from build123d import *

# Parameters (mm, degrees)
BOSS_EXTRU_7_DEPTH          = 35
BOSS_EXTRU_8_DEPTH          = 5
ESQUISSE3_R                 = 2.5
ENL_V_MAT_EXTRU_1_DEPTH     = 5
ENL_V_MAT_EXTRU_2_DEPTH     = 12
ESQUISSE6_R                 = 9.75
ENL_V_MAT_EXTRU_3_DEPTH     = 5
CONG_1_R                    = 2
ESQUISSE8_R                 = 1.5
ENL_V_MAT_EXTRU_5_DEPTH     = 90.727364834
TROU_TARAUD_M31_D           = 2.5
TROU_TARAUD_M31_DEPTH       = 12.5
TROU_TARAUD_M31_TIP         = 0.751075774
ENL_V_START                 = -35
ENL_V_MAT_EXTRU_6_OUTLINE_R = 1.475
ENL_V_MAT_EXTRU_6_DEPTH     = 10
ENL_V_MAT_EXTRU_7_DEPTH     = 99.692704898
ENL_V_MAT_EXTRU_8_DEPTH     = 10


# Read off the part's stored shape, not the designer's step: Enlèv. mat.-Extru.6
with BuildPart() as part:
    # Esquisse1 → Boss.-Extru.7 (new, symmetric)
    with BuildSketch(Plane(origin=(0, 0, 0), x_dir=(1, 0, 0), z_dir=(0, 1, 0))):
        Polygon((-35, 31), (-35, -31), (0, -31), (0, -26), (-25, -26), (-25, -22.1), (-25, -17.1), (-25, 17.1), (-25, 22.1), (-25, 26), (0, 26), (0, 31), align=None)
    extrude(amount=BOSS_EXTRU_7_DEPTH, both=True)

    # Esquisse2 → Boss.-Extru.8 (add)
    with BuildSketch(Plane.XZ.offset(35)):
        with BuildLine():
            Line((-35, 37.094473982), (-35, -37.094473982))
            ThreePointArc((-35, -37.094473982), (-18.830584523, -47.396298237), (0, -51))
            Line((0, -51), (0, 51))
            ThreePointArc((0, 51), (-18.830584523, 47.396298237), (-35, 37.094473982))
        make_face()
    extrude(amount=-BOSS_EXTRU_8_DEPTH)

    # Esquisse3 → Enlèv. mat.-Extru.1 (cut)
    with BuildSketch(Plane(origin=(-25, 0, 0), x_dir=(0, 0, -1), z_dir=(1, 0, 0))):
        with Locations((-19.6, -2.21)):
            Circle(ESQUISSE3_R)
        with Locations((19.6, -2.21)):
            Circle(ESQUISSE3_R)
    extrude(amount=-ENL_V_MAT_EXTRU_1_DEPTH, mode=Mode.SUBTRACT)

    # Esquisse5 → Enlèv. mat.-Extru.2 (cut)
    with BuildSketch(Plane(origin=(0, 0, 0), x_dir=(0, 0, -1), z_dir=(1, 0, 0))):
        with BuildLine():
            Line((98.051206934, 14.815086571), (40.674477228, 51.032394683))
            ThreePointArc((40.674477228, 51.032394683), (34.260412481, 48.633219758), (27.706013605, 46.649253461))
            ThreePointArc((27.706013605, 46.649253461), (-0.631861598, 43.001865666), (-28.924683694, 46.983677637))
            ThreePointArc((-28.924683694, 46.983677637), (-34.858411147, 48.837303455), (-40.674477228, 51.032394683))
            Line((-40.674477228, 51.032394683), (-98.051206934, 14.815086571))
            ThreePointArc((-98.051206934, 14.815086571), (-66.125172065, -3.350779651), (-31, -14.097531974))
            Line((-31, -14.097531974), (-31, 35))
            Line((-31, 35), (-26, 35))
            Line((-26, 35), (-26, -14.963632356))
            ThreePointArc((-26, -14.963632356), (0, -17), (26, -14.963632356))
            Line((26, -14.963632356), (26, 35))
            Line((26, 35), (31, 35))
            Line((31, 35), (31, -14.097531974))
            ThreePointArc((31, -14.097531974), (66.125172065, -3.350779651), (98.051206934, 14.815086571))
        make_face()
        with BuildLine():
            ThreePointArc((-31, -14.097531974), (-28.503289853, -14.549574498), (-26, -14.963632356))
            Line((-26, -14.963632356), (-26, 35))
            Line((-26, 35), (-31, 35))
            Line((-31, 35), (-31, -14.097531974))
        make_face()
        with BuildLine():
            ThreePointArc((26, -14.963632356), (28.503289853, -14.549574498), (31, -14.097531974))
            Line((31, -14.097531974), (31, 35))
            Line((31, 35), (26, 35))
            Line((26, 35), (26, -14.963632356))
        make_face()
    extrude(amount=-ENL_V_MAT_EXTRU_2_DEPTH, mode=Mode.SUBTRACT)

    # Esquisse6 → Enlèv. mat.-Extru.3 (cut)
    with BuildSketch(Plane(origin=(-25, 0, 0), x_dir=(0, 0, -1), z_dir=(1, 0, 0))):
        with Locations((0, 20)):
            Circle(ESQUISSE6_R)
    extrude(amount=-ENL_V_MAT_EXTRU_3_DEPTH, mode=Mode.SUBTRACT)

    # Congé1
    cong_1_edges = [part.edges().sort_by_distance(p)[0] for p in [
        (-23.5, 35, 31),
        (-18.5, 35, 26),
        (-25, 35, 0),
        (-18.5, 35, -26),
        (-23.5, 35, -31),
        (-12, 35, -28.5),
        (-12, 35, 28.5),
        (-35, 35, 0),
    ]]
    fillet(cong_1_edges, radius=CONG_1_R)

    # Esquisse8 → Enlèv. mat.-Extru.5 (cut, through all)
    with BuildSketch(Plane(origin=(0, -30, 0), x_dir=(1, 0, 0), z_dir=(0, 1, 0))):
        with Locations(Location((-21, 41, 0), (0, 0, 270))):
            Circle(ESQUISSE8_R)
        with Locations(Location((-6, 41, 0), (0, 0, 270))):
            Circle(ESQUISSE8_R)
        with Locations(Location((-6, -41, 0), (0, 0, 90))):
            Circle(ESQUISSE8_R)
        with Locations(Location((-21, -41, 0), (0, 0, 90))):
            Circle(ESQUISSE8_R)
    extrude(amount=-ENL_V_MAT_EXTRU_5_DEPTH, mode=Mode.SUBTRACT)

    # Trou taraudé M31
    with Locations(Plane(origin=(-35, 18, -4), x_dir=(0, 0, -1), z_dir=(-1, 0, 0))):
        with Locations((0, 0), (-15, 0), (-30, 0)):
            Hole(TROU_TARAUD_M31_D / 2, depth=TROU_TARAUD_M31_DEPTH)
            with Locations((0, 0, -(TROU_TARAUD_M31_DEPTH + TROU_TARAUD_M31_TIP / 2))):  # 118° drill point
                Cone(0, TROU_TARAUD_M31_D / 2, TROU_TARAUD_M31_TIP, mode=Mode.SUBTRACT)

    # Enlèv. mat.-Extru.6 outline → Enlèv. mat.-Extru.6 (cut)
    with BuildSketch(Plane.YZ.offset(ENL_V_START)):
        with Locations((10, -14.5)):
            Circle(ENL_V_MAT_EXTRU_6_OUTLINE_R)
        with Locations((10, 14.5)):
            Circle(ENL_V_MAT_EXTRU_6_OUTLINE_R)
    extrude(amount=ENL_V_MAT_EXTRU_6_DEPTH, mode=Mode.SUBTRACT)

    # Esquisse3D3 → Enlèv. mat.-Extru.7 (cut, through all)
    with BuildSketch(Plane(origin=(0, -30, -14.5), x_dir=(-0.586509812151843, 0, 0.8099421215430211), z_dir=(0, -1, 0))):
        Polygon((0, 0), (12.316706055, 17.008784552), (35.80502758, 0), (23.488321525, -17.008784552), align=None)
    extrude(amount=ENL_V_MAT_EXTRU_7_DEPTH, mode=Mode.SUBTRACT)

    # Esquisse3D4 → Enlèv. mat.-Extru.8 (cut)
    with BuildSketch(Plane(origin=(0, -22, -31), x_dir=(-0.8574929257125444, -0.5144957554275261, 0), z_dir=(0, 0, -1))):
        Polygon((0, 0), (4.287464629, 2.572478777), (5.830951895, 0), (1.543487266, -2.572478777), align=None)
    extrude(amount=-ENL_V_MAT_EXTRU_8_DEPTH, mode=Mode.SUBTRACT)


solid = part.part
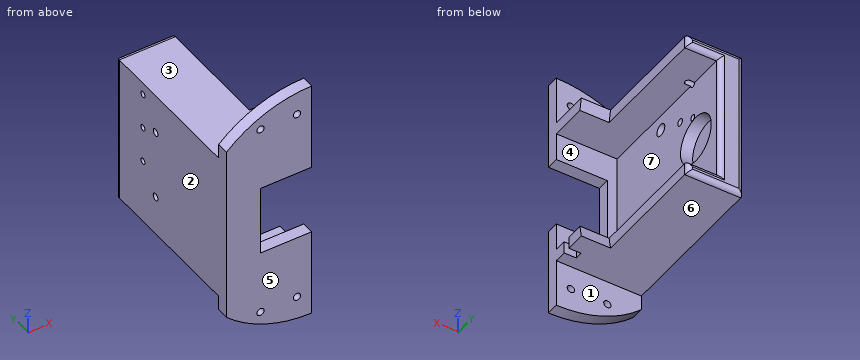
Design review of the part built by this model. Coordinates are the model's own, in mm. Face numbers are marked on the shaded views. A direction names the side the tool comes from. Coordinates: 2 decimals unless noted, no trailing zeros. Loops run counter-clockwise (first coordinate to the right, second up) from the corner with the lowest first, then second, coordinate; pieces in that order, holes last.
Item 1: For the marked faces 1, 2, 3 and 4, list the 3-axis set-ups (+Z, -Z, +X, -X, +Y, -Y) from which the entire face can be reached by the end or side of a thin tool; tool diameter is ignored.
Completed:
face 1: -Z, +X, -X, +Y
face 2: +Z, -Z, -X, +Y, -Y
face 3: +Z, +X, -X, +Y
face 4: +X, +Y
Item 2: Clearance check with flat-ended pins moving along their axes: pin 1 (4 mm diameter, centred on x = -6, z = -41, fed in from +Y); pin 2 (2.5 mm diameter, centred on x = -2, z = -28.5, fed in from +Y); pin 3 (2.5 mm diameter, centred on y = -2.5, z = 19, fed in from +X). State where each tip first meets the part, or that it passes through.
Completed:
pin 1: stops at y = -30
pin 2: stops at y = -14.33
pin 3: stops at x = -30
Item 3: Wall thickness on L1, parallel to Y at x = -28.6, z = 0; L2, parallel to Z at x = -24, y = 18; L3, parallel to Z at x = -32, y = 18: over which ranges is each line inside the solid? List them lowest first.
Completed:
L1: y = -35 to 10.25, 29.75 to 35
L2: z = -31 to -26, 27.25 to 31
L3: z = -31 to -5.25, -2.75 to 9.75, 12.25 to 24.75, 27.25 to 31
Item 4: Add section C-C (z = 41). Write out the cut boundary in (x, y).
Completed:
outline: (-30.33, -35) - (-22.5, -35) - (-22.5, -30) - (-30.33, -30) - close; (-19.5, -35) - (-7.5, -35) - (-7.5, -30) - (-19.5, -30) - close; (-4.5, -35) - (0, -35) - (0, -30) - (-4.5, -30) - close
Item 5: Add section B-B (z = -19.6). Write out the cut boundary in (x, y).
Completed:
outline: (-35, -35) - (0, -35) - (0, -30) - (-25, -30) - (-25, -4.71) - (-30, -4.71) - (-30, 0.29) - (-25, 0.29) - (-25, 33) arc R2 ccw to (-27, 35) - (-33, 35) arc R2 ccw to (-35, 33) - close
Item 6: Add section A-A (y = -8.5). Write out the cut boundary in (x, z).
Completed:
outline: (-35, -31) - (-12, -31) - (-12, -26) - (-25, -26) - (-25, 26) - (-12, 26) - (-12, 31) - (-35, 31) - close
Item 7: Add section D-D (y = 15). Write out the cut boundary in (x, z), and give its area (3 significant figures).
Completed:
outline: (-35, -31) - (-12, -31) - (-12, -26) - (-25, -26) - (-25, -8.37) - (-30, -8.37) - (-30, 8.37) - (-25, 8.37) - (-25, 26) - (-12, 26) - (-12, 31) - (-35, 31) - close
area: 666 mm2
Item 8: Draft analysis for pull direction Z (two halves, no side actions). For the marked faces 5, 6 and 7, state which applies: pulls with the +Z half, pulls with the -Z half, needs draft (parallel to the pull), parting line crosses it, or undercut.
Completed:
face 5: needs draft
face 6: pulls with the -Z half
face 7: undercut
